Read the model definition and answer for the solid it produces. Units are mm, in the model's axes. Face numbers are marked on the shaded views. A direction names the side the tool comes from. Coordinates: 2 decimals unless noted, no trailing zeros. Write each loop counter-clockwise with the first axis right and the second up, starting at its lowest first coordinate (ties: lowest second). Pieces come first, ordered by that corner, then holes. Notation, with made-up numbers: (-13, 37.5) - (-7, 37.5) arc R30 cw to (-7, 72.5) - close; hole circle Ø6 at (-23, -14). An arc over 180 degrees is marked (long way). Use a Markdown table: item, result.
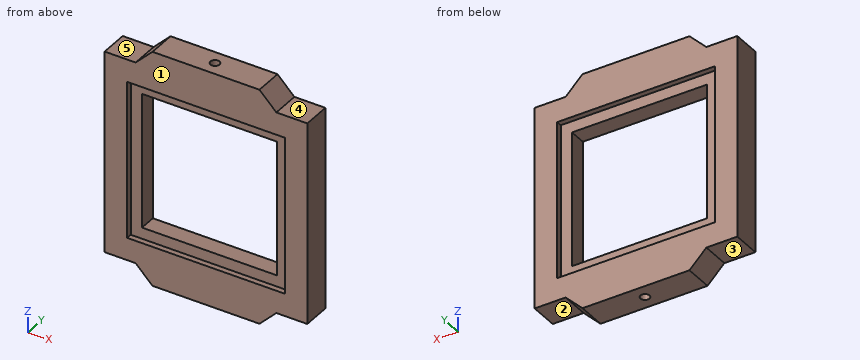
from build123d import *

# Parameters (mm, degrees)
F0_W      = 180
F0_H      = 180
F1_DEPTH  = 25
F2_W      = 125
F2_H      = 25
F3_DEPTH  = 15
F4_W      = 125
F4_H      = 25
F5_DEPTH  = 15
F7_DEPTH  = 25
F8_W      = 120
F8_H      = 120
F9_DEPTH  = 25
F10_W     = 140
F10_H     = 140
F11_DEPTH = 5
F12_W     = 140
F12_H     = 140
F13_DEPTH = 5
F14_R     = 4
F15_DEPTH = 25
F16_R     = 4
F17_DEPTH = 25


with BuildPart() as f1:
    # F0 (on Front) → F1 (new body)
    with BuildSketch(Plane.XZ):
        Rectangle(F0_W, F0_H)
    extrude(amount=F1_DEPTH)

    # F2 (on face) → F3 (join)
    with BuildSketch(Plane(origin=(0, 0, -90), x_dir=(1, 0, 0), z_dir=(0, 0, -1))):
        with Locations((0, 12.5)):
            Rectangle(F2_W, F2_H)
    extrude(amount=F3_DEPTH)

    # F4 (on face) → F5 (join)
    with BuildSketch(Plane.XY.offset(90)):
        with Locations((0, -12.5)):
            Rectangle(F4_W, F4_H)
    extrude(amount=F5_DEPTH)

    # F6 (on face) → F7 (cut)
    with BuildSketch(Plane.XZ.offset(25)):
        Polygon((-47.5, -105), (-62.5, -90), (-62.5, -105), align=None)
        Polygon((62.5, -105), (62.5, -90), (47.5, -105), align=None)
        Polygon((-62.5, 105), (-62.5, 90), (-47.5, 105), align=None)
        Polygon((47.5, 105), (62.5, 90), (62.5, 105), align=None)
    extrude(amount=-F7_DEPTH, mode=Mode.SUBTRACT)

    # F8 (on face) → F9 (cut)
    with BuildSketch(Plane(origin=(0, 0, 0), x_dir=(-1, 0, 0), z_dir=(0, 1, 0))):
        Rectangle(F8_W, F8_H)
    extrude(amount=-F9_DEPTH, mode=Mode.SUBTRACT)

    # F10 (on face) → F11 (cut)
    with BuildSketch(Plane(origin=(0, 0, 0), x_dir=(-1, 0, 0), z_dir=(0, 1, 0))):
        Rectangle(F10_W, F10_H)
    extrude(amount=-F11_DEPTH, mode=Mode.SUBTRACT)

    # F12 (on face) → F13 (cut)
    with BuildSketch(Plane.XZ.offset(25)):
        Rectangle(F12_W, F12_H)
    extrude(amount=-F13_DEPTH, mode=Mode.SUBTRACT)

    # F14 (on face) → F15 (cut)
    with BuildSketch(Plane(origin=(0, 0, -105), x_dir=(1, 0, 0), z_dir=(0, 0, -1))):
        with Locations((0, 12.5)):
            Circle(F14_R)
    extrude(amount=-F15_DEPTH, mode=Mode.SUBTRACT)

    # F16 (on face) → F17 (cut)
    with BuildSketch(Plane.XY.offset(105)):
        with Locations((0, -12.5)):
            Circle(F16_R)
    extrude(amount=-F17_DEPTH, mode=Mode.SUBTRACT)


solid = f1.part
(1) A cutting plane is placed at C-C, the plane z = -4. Write down the section's boundary in (x, y).
Report:
| item | result |
|---|---|
| outline | (-90, -25) - (-70, -25) - (-70, -20) - (-60, -20) - (-60, -5) - (-70, -5) - (-70, 0) - (-90, 0) - close; (60, -20) - (70, -20) - (70, -25) - (90, -25) - (90, 0) - (70, 0) - (70, -5) - (60, -5) - close |
(2) Straight lines are drawn through the part: L1, parallel to X at y = -12.5, z = -87.75; L2, parallel to Y at x = 0, z = 99; L3, parallel to Z at x = 34, y = -8.75. For each, find the intervals that lie inside material, in ascending order.
Report:
| item | result |
|---|---|
| L1 | x = -90 to -4, 4 to 90 |
| L2 | y = -25 to -16.5, -8.5 to 0 |
| L3 | z = -105 to -60, 60 to 105 |
(3) For the marked faces 1, 2, 3, 4 and 5, determine the directions among +Z, -Z, +X, -X, +Y, -Y from which every point of the face is accessible in a straight line to the end or side of a thin tool.
Report:
| item | result |
|---|---|
| face 1 | +Z, -Z, +X, -X, -Y |
| face 2 | -Z, +X, +Y, -Y |
| face 3 | -Z, -X, +Y, -Y |
| face 4 | +Z, +X, +Y, -Y |
| face 5 | +Z, -X, +Y, -Y |
(4) A cutting plane is placed at B-B, the plane y = -2.75. Write down the section's boundary in (x, z).
Report:
| item | result |
|---|---|
| outline | (-90, -90) - (-62.5, -90) - (-47.5, -105) - (47.5, -105) - (62.5, -90) - (90, -90) - (90, 90) - (62.5, 90) - (47.5, 105) - (-47.5, 105) - (-62.5, 90) - (-90, 90) - close; hole (-70, -70) - (70, -70) - (70, 70) - (-70, 70) - close |
(5) Each of these flat-tipped pins is pushed along its axis until it touches: P1, Ø1, axis at x = -69.5, y = -4.5, coming from the +Z side; P2, Ø3, axis at x = 50.5, y = -5.5, coming from the -Z side. Where does it stop, or does it pass through?
Report:
| item | result |
|---|---|
| P1 | stops at z = 90 |
| P2 | stops at z = -103.5 |
(6) A cutting plane is placed at D-D, the plane x = 23. Write down the section's boundary in (y, z), and give its area (3 significant figures).
Report:
| item | result |
|---|---|
| outline | (-25, -105) - (0, -105) - (0, -70) - (-5, -70) - (-5, -60) - (-20, -60) - (-20, -70) - (-25, -70) - close; (-25, 70) - (-20, 70) - (-20, 60) - (-5, 60) - (-5, 70) - (0, 70) - (0, 105) - (-25, 105) - close |
| area | 2,050 mm² |
(7) A cutting plane is placed at A-A, the plane x = 0. Write down the section's boundary in (y, z), and give its area (3 significant figures).
Report:
| item | result |
|---|---|
| outline | (-25, -105) - (-16.5, -105) - (-16.5, -80) - (-8.5, -80) - (-8.5, -105) - (0, -105) - (0, -70) - (-5, -70) - (-5, -60) - (-20, -60) - (-20, -70) - (-25, -70) - close; (-25, 70) - (-20, 70) - (-20, 60) - (-5, 60) - (-5, 70) - (0, 70) - (0, 105) - (-8.5, 105) - (-8.5, 80) - (-16.5, 80) - (-16.5, 105) - (-25, 105) - close |
| area | 1,650 mm² |
